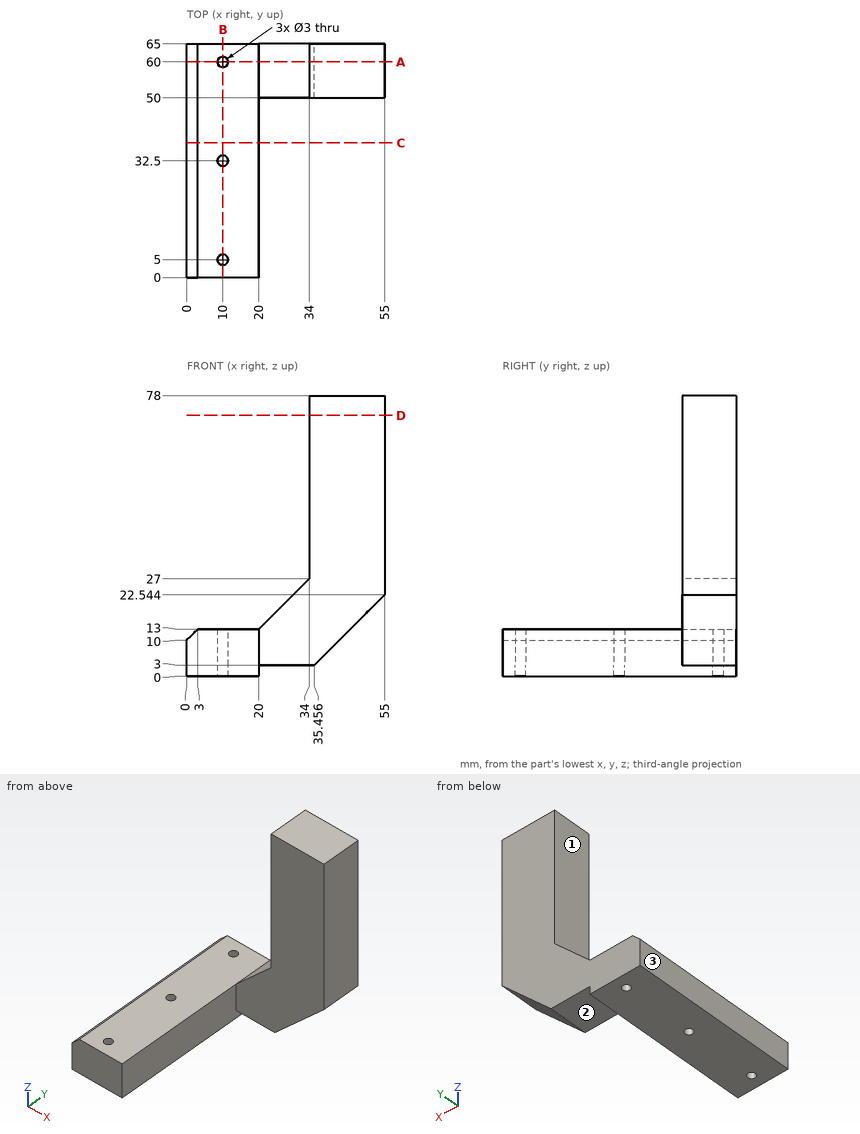
The figure shows three views and two pictorial views of one solid part (mm, origin at its lowest corner). Answer the questions. A direction names the side the tool comes from. Coordinates: 2 decimals unless noted, no trailing zeros. Loops run counter-clockwise (first coordinate to the right, second up) from the corner with the lowest first, then second, coordinate; pieces in that order, holes last.
(1) Consider line 1 along Y through (x, z) = (10, 10.5); line 2 along X through (y, z) = (5, 7); line 3 along Z through (x, y) = (9, 57.5). Determine where each line is inside the solid, lowest interval first.
Solution:
line 1: y = 0 to 3.5, 6.5 to 31, 34 to 58.5, 61.5 to 65
line 2: x = 0 to 8.5, 11.5 to 20
line 3: z = 0 to 13
(2) The part is cut by section B-B (x = 10). Determine the outline of the cut face in (y, z), and give its area (3 significant figures).
Solution:
outline: (0, 0) - (3.5, 0) - (3.5, 13) - (0, 13) - close; (6.5, 0) - (31, 0) - (31, 13) - (6.5, 13) - close; (34, 0) - (58.5, 0) - (58.5, 13) - (34, 13) - close; (61.5, 0) - (65, 0) - (65, 13) - (61.5, 13) - close
area: 728 mm2
(3) The part is cut by section A-A (y = 60). Determine the outline of the cut face in (x, z), and give its area (3 significant figures).
Solution:
outline: (0, 0) - (8.5, 0) - (8.5, 13) - (3, 13) - (0, 10) - close; (11.5, 0) - (20, 0) - (20, 3) - (35.46, 3) - (55, 22.54) - (55, 78) - (34, 78) - (34, 27) - (20, 13) - (11.5, 13) - close
area: 1,840 mm2
(4) The part is cut by section C-C (y = 37.5). Determine the outline of the cut face in (x, z), and give its area (4 significant figures).
Solution:
outline: (0, 0) - (20, 0) - (20, 13) - (3, 13) - (0, 10) - close
area: 255.5 mm2
(5) The part is cut by section D-D (z = 72.5). Determine the outline of the cut face in (x, y), and give its area (3 significant figures).
Solution:
outline: (34, 50) - (55, 50) - (55, 65) - (34, 65) - close
area: 315 mm2
(6) A tool of negligible diameter and unlimited length cuts with its end or side. For the marked faces 1, 2 and 3, from which of +Z, -Z, +X, -X, +Y, -Y can it reach the whole face along a straight path? Write none if from no direction.
Solution:
face 1: +Z, -X, +Y, -Y
face 2: -Z, +X, +Y, -Y
face 3: +Z, -Z, -X, +Y, -Y
(7) Flat-ended cylindrical pins translate along their axes: pin 1 Ø3.5 at (x, y) = (10, 32.5) entering from +Z; pin 2 Ø12 at (x, y) = (29.5, 60) entering from -Z; pin 3 Ø10.5 at (x, z) = (34, 50) entering from -Y. Find the tip coordinate at first contact, or state that the pin passes through.
Solution:
pin 1: stops at z = 13
pin 2: stops at z = 3
pin 3: stops at y = 50
